```python
from build123d import *

# Parameters (mm, degrees)
F1_DEPTH = 698.5
F3_DEPTH = 19.05
F5_DEPTH = 19.05
F6_W     = 260.35
F6_H     = 15.875
F7_DEPTH = 266.7


with BuildPart() as f1:
    # F0 (on Top) → F1 (new body)
    with BuildSketch(Plane.XY):
        Polygon((-133.35, -136.525), (-133.35, 136.525), (133.35, 136.525), (133.35, -136.525), (114.3, -136.525), (114.3, -155.575), (152.4, -155.575), (152.4, 155.575), (-152.4, 155.575), (-152.4, -155.575), (-114.3, -155.575), (-114.3, -136.525), align=None)
    extrude(amount=F1_DEPTH)

    # F2 (on face) → F3 (join)
    with BuildSketch(Plane.XY.offset(698.5)):
        Polygon((152.4, 155.575), (-152.4, 155.575), (-152.4, -155.575), (-114.3, -155.575), (-114.3, -136.525), (-133.35, -136.525), (-133.35, 136.525), (133.35, 136.525), (133.35, -136.525), (114.3, -136.525), (114.3, -155.575), (152.4, -155.575), align=None)
        Polygon((-114.3, -136.525), (-114.3, -155.575), (114.3, -155.575), (114.3, -136.525), (133.35, -136.525), (133.35, 136.525), (-133.35, 136.525), (-133.35, -136.525), align=None)
    extrude(amount=F3_DEPTH)

    # F4 (on face) → F5 (join)
    with BuildSketch(Plane(origin=(0, 0, 0), x_dir=(1, 0, 0), z_dir=(0, 0, -1))):
        Polygon((114.3, 155.575), (-114.3, 155.575), (-114.3, 136.525), (-133.35, 136.525), (-133.35, -136.525), (133.35, -136.525), (133.35, 136.525), (114.3, 136.525), align=None)
        Polygon((-152.4, 155.575), (-152.4, -155.575), (152.4, -155.575), (152.4, 155.575), (114.3, 155.575), (114.3, 136.525), (133.35, 136.525), (133.35, -136.525), (-133.35, -136.525), (-133.35, 136.525), (-114.3, 136.525), (-114.3, 155.575), align=None)
    extrude(amount=F5_DEPTH)

    # F6 (on face) → F7 (join, through all)
    with BuildSketch(Plane.YZ.offset(-133.35)):
        with Locations((0, 493.7125)):
            Rectangle(F6_W, F6_H)
        with Locations((0, 236.5375)):
            Rectangle(F6_W, F6_H)
    extrude(amount=F7_DEPTH)


solid = f1.part
```
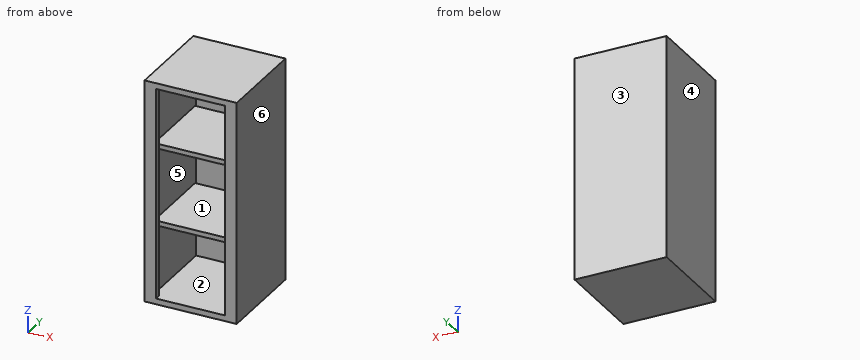
Check sheet for the modelled part. Datum: model origin and axes. Units: mm. Face numbers are marked on the shaded views. A direction names the side the tool comes from. Round coordinates to 2 decimals unless told otherwise and drop trailing zeros. Loops run counter-clockwise (first coordinate to the right, second up) from the corner with the lowest first, then second, coordinate; pieces in that order, holes last. Notation, with made-up numbers: (54, -6.5) - (84, -6.5) arc R23 ccw to (84, 32.5) - close; hole circle Ø1 at (12.5, -8.5). An arc over 180 degrees is marked (long way). Write item = value, one per line. Start each with the question number.
Q1. Access from +Z, -Z, +X, -X, +Y, -Y to the whole of each face (thin tool, end or side, straight path). Record for the marked faces 5 and 6.
Q2. Release check for a two-part mould opening along X. For the marked faces 1, 2, 3 and 4 record: pulls with the +X half, pulls with the -X half, needs draft (parallel to the pull), parting line crosses it, or undercut.
Q3. Thickness scan on L1, parallel to Z at x = -24.5, y = -17 (3 decimals); L2, parallel to X at y = 23, z = 365; L3, parallel to Z at x = -106, y = -137.5. Record the ranges inside material, lowest first.
Q4. Section check C-C (z = 218.5). Record the boundary of the cut face in (x, y) (3 decimals).
Q5. Depth check by flat-ended pin: P1, Ø10, axis at x = 46, z = 224.5, coming from the -Y side (3 decimals). Enter the tip coordinate at first touch or a pass-through.
Q6. Section check B-B (y = 113.5). Record the boundary of the cut face in (x, z) (3 decimals), plus the area to 3 significant figures.
Q7. Section check A-A (x = -19). Record the boundary of the cut face in (y, z) (3 decimals).
Derived:
q1.face_5 = none
q1.face_6 = +Z, -Z, +X, +Y, -Y
q2.face_1 = undercut
q2.face_2 = undercut
q2.face_3 = needs draft
q2.face_4 = pulls with the -X half
q3.L1 = -19.05 to 0, 228.6 to 244.475, 485.775 to 501.65, 698.5 to 717.55
q3.L2 = -152.4 to -133.35, 133.35 to 152.4
q3.L3 = -19.05 to 0, 698.5 to 717.55
q4.outline = (-152.4, -155.575) - (-114.3, -155.575) - (-114.3, -136.525) - (-133.35, -136.525) - (-133.35, 136.525) - (133.35, 136.525) - (133.35, -136.525) - (114.3, -136.525) - (114.3, -155.575) - (152.4, -155.575) - (152.4, 155.575) - (-152.4, 155.575) - close
q5.P1 = -130.175
q6.outline = (-152.4, -19.05) - (152.4, -19.05) - (152.4, 717.55) - (-152.4, 717.55) - close; hole (-133.35, 0) - (133.35, 0) - (133.35, 228.6) - (-133.35, 228.6) - close; hole (-133.35, 244.475) - (133.35, 244.475) - (133.35, 485.775) - (-133.35, 485.775) - close; hole (-133.35, 501.65) - (133.35, 501.65) - (133.35, 698.5) - (-133.35, 698.5) - close
q6.area = 46,700 mm^2
q7.outline = (-155.575, -19.05) - (155.575, -19.05) - (155.575, 717.55) - (-155.575, 717.55) - (-155.575, 698.5) - (136.525, 698.5) - (136.525, 0) - (-155.575, 0) - close; (-130.175, 228.6) - (130.175, 228.6) - (130.175, 244.475) - (-130.175, 244.475) - close; (-130.175, 485.775) - (130.175, 485.775) - (130.175, 501.65) - (-130.175, 501.65) - close
